For this review, use the dimensioned drawing (mm, ordinates from the lowest corner) and the shaded views. A direction names the side the tool comes from. Round coordinates to 2 decimals unless told otherwise and drop trailing zeros. Order: outer loops, then holes, each group sorted by start corner. A loop starts at its lowest first (then second) coordinate and runs counter-clockwise, first axis right, second up. Notation, with made-up numbers: (74.5, 50) -> (92.5, 50) arc R25 ccw to (92.5, 86) -> close; hole circle Ø8 at (66.25, 68). An arc over 180 degrees is marked (long way). Use a Markdown table: item, result. Add a question column.
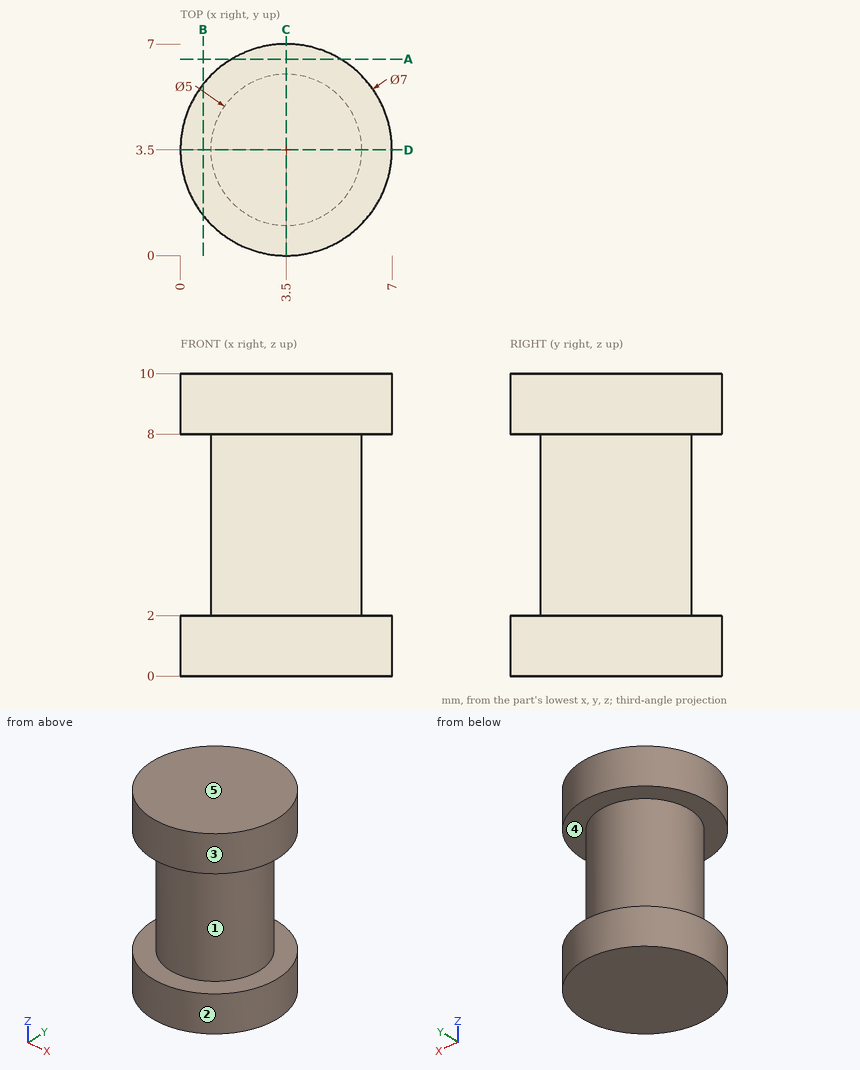
Q1. Add section A-A (y = 6.5). Write out the cut boundary in (x, z), then the cut area to 3 significant figures.
Q2. Add section B-B (x = 0.75). Write out the cut boundary in (y, z).
Q3. Insertion check: pin 1 (1 mm diameter, centred on x = 4, z = 5, fed in from +Y); pin 2 (1.5 mm diameter, centred on x = 1.5, z = 8.5, fed in from +Y); pin 3 (1.5 mm diameter, centred on y = 6, z = 5, fed in from -X). Each pin has a flat end and moves straight along its axis. Give the tip position at first contact, or say it passes through.
Q4. Add section C-C (x = 3.5). Write out the cut boundary in (y, z).
Q5. Machinability: for the marked faces 1 and 2, which of the approach directions +Z, -Z, +X, -X, +Y, -Y give a long, thin tool a straight path to every point of the face, cutting with its end or side? Answer none if there is none.
Q6. Mouldability with a two-part tool opening along Z and no side actions: class the marked faces 3, 4 and 5 as pulls with the +Z half, pulls with the -Z half, needs draft (parallel to the pull), parting line crosses it, or undercut.
Q7. Wall thickness on line 1 (Z direction, x = 5.75, y = 2); line 2 (Y direction, x = 5.75, z = 0.75); line 3 (X direction, y = 5.75, z = 3): over which ranges is each line inside the solid? List them lowest first. Write a range as [from, to].
Report:
| question | item | result |
|---|---|---|
| 1 | outline | (1.7, 0) -> (5.3, 0) -> (5.3, 2) -> (1.7, 2) -> close; (1.7, 8) -> (5.3, 8) -> (5.3, 10) -> (1.7, 10) -> close |
| 1 | area | 14.4 mm² |
| 2 | outline | (1.33, 0) -> (5.67, 0) -> (5.67, 2) -> (1.33, 2) -> close; (1.33, 8) -> (5.67, 8) -> (5.67, 10) -> (1.33, 10) -> close |
| 3 | pin 1 | stops at y = 6 |
| 3 | pin 2 | stops at y = 6.77 |
| 3 | pin 3 | stops at x = 1.71 |
| 4 | outline | (0, 0) -> (7, 0) -> (7, 2) -> (6, 2) -> (6, 8) -> (7, 8) -> (7, 10) -> (0, 10) -> (0, 8) -> (1, 8) -> (1, 2) -> (0, 2) -> close |
| 5 | face 1 | none |
| 5 | face 2 | +Z, -Z |
| 6 | face 3 | needs draft |
| 6 | face 4 | undercut |
| 6 | face 5 | pulls with the +Z half |
| 7 | line 1 | z = [0, 2], [8, 10] |
| 7 | line 2 | y = [0.82, 6.18] |
| 7 | line 3 | x = [2.41, 4.59] |
